Geometry check sheet. Reference: the model listing, model coordinates, mm. Face numbers are marked on the shaded views. Give positions to 0.01 mm unless a question says otherwise; leave off trailing zeros. Order: outer loops, then holes, each group sorted by start corner. A loop starts at its lowest first (then second) coordinate and runs counter-clockwise, first axis right, second up. Notation, with made-up numbers: M -24.75,24 L 23.25,24 A22 ccw 23.25,55 Z; hole C 11.25,59 d9. An arc over 180 degrees is marked long. Answer as CSV lines item,"result". Start each with the question number.
Q1. Section check A-A, the plane y = 2.7. Record the boundary of the cut face in (x, z).
Q2. Mould release check, pull along X, two halves, no side actions. Record for the marked faces 1, 2, 3 and 4: +X half, -X half, draft (parallel to the pull), parting line (faces both ways), or undercut.
Q3. Thickness scan on line 1 (X direction, y = 2.4, z = 0); line 2 (X direction, y = 2.3, z = 0); line 3 (Y direction, x = -30, z = -1.25). Record the ranges inside material, lowest first.
Q4. Section check C-C, the plane z = 0. Record the boundary of the cut face in (x, y), then the cut area to 3 significant figures.
Q5. Section check B-B, the plane x = 0. Record the boundary of the cut face in (y, z), then the cut area to 3 significant figures.
Q6. Section check D-D, the plane x = 11.5. Record the boundary of the cut face in (y, z), then the cut area to 3 significant figures.
Q7. Go/stop test with flat-tipped pins: pin 1 (1 mm diameter, centred on x = 23.5, y = 1.5, fed in from -Z); pin 2 (5 mm diameter, centred on x = 28, z = 0, fed in from -Y); pin 3 (16 mm diameter, centred on x = 0, z = 0, fed in from -Y). Record where each tip stops, or that it passes through.
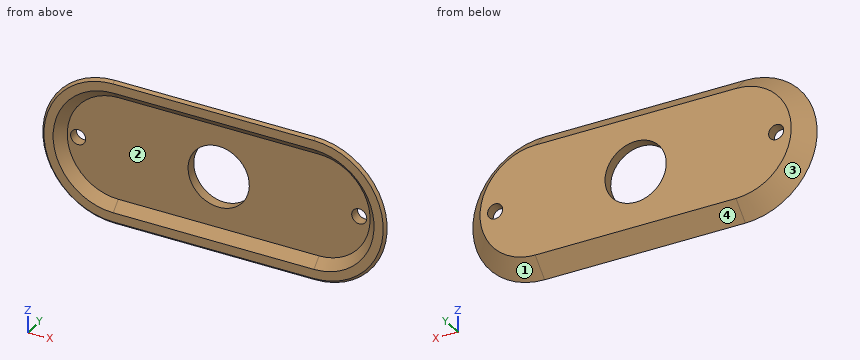
```python
from build123d import *
from OCP.BRepFilletAPI import BRepFilletAPI_MakeChamfer

# Parameters (mm, degrees)
BOSS_EXTRU_1_DEPTH      = 3.8
BOSS_EXTRU_1_TAPER      = 45
COQUE2_DEPTH            = 1.8
COQUE2_DRAFT            = 45
CHANFREIN1_SIZE         = 1
CHANFREIN1_SIZE2        = 0.707106781
ENL_V_MAT_EXTRU_1_REACH = 39.355
ESQUISSE2_R             = 1.5
ENL_V_MAT_EXTRU_2_REACH = 39.215
ESQUISSE3_R             = 6.1


# Read off the part's stored shape, not the designer's step: Coque2
with BuildPart() as part:
    # Esquisse1 → Boss.-Extru.1 (new body)
    with BuildSketch(Plane(origin=(0, 0, 0), x_dir=(1, 0, 0), z_dir=(0, 1, 0))):
        with BuildLine():
            ThreePointArc((-20, 14.8), (-34.8, 0), (-20, -14.8))
            Line((-20, -14.8), (20, -14.8))
            ThreePointArc((20, -14.8), (34.8, 0), (20, 14.8))
            Line((20, 14.8), (-20, 14.8))
        make_face()
    extrude(amount=BOSS_EXTRU_1_DEPTH, taper=BOSS_EXTRU_1_TAPER)


with BuildPart() as coque2_tool:
    # Coque2 outline → Coque2 (with draft: the straight prism first)
    with BuildSketch(Plane(origin=(0, 1.8, 0), x_dir=(1, 0, 0), z_dir=(0, 1, 0))):
        with BuildLine():
            Line((-20, -10.171572875), (20, -10.171572875))
            ThreePointArc((20, -10.171572875), (30.171572875, 0), (20, 10.171572875))
            Line((20, 10.171572875), (-20, 10.171572875))
            ThreePointArc((-20, 10.171572875), (-30.171572875, 0), (-20, -10.171572875))
        make_face()
    extrude(amount=-COQUE2_DEPTH)
    # Coque2: the draft: its side faces are tilted about the plane it starts from
    coque2_sides = [coque2_tool.faces().sort_by_distance(p)[0] for p in [
        (0, 0.9, 10.171572875),
        (30.171572875, 0.9, 0),
        (0, 0.9, -10.171572875),
        (-30.171572875, 0.9, 0),
    ]]
    draft(coque2_sides, Plane(origin=(0, 1.8, 0), x_dir=(1, 0, 0), z_dir=(0, 1, 0)), COQUE2_DRAFT)


with BuildPart() as part_1:
    add(part.part)

    # Coque2: cut by coque2_tool
    add(coque2_tool.part, mode=Mode.SUBTRACT)

    # Chanfrein1: one chamfer whose edges measure the first distance from different faces: ONE call of the kernel's chamfer builder (chamfer() names one face for all edges)
    chanfrein1_edges_1 = [part_1.edges().sort_by_distance(p)[0] for p in [
        (0, 0, -14.8),
        (0, 0, 14.8),
        (-34.8, 0, 0),
    ]]
    chanfrein1_side_1 = [part_1.faces().sort_by_distance(p)[0] for p in [
        (0, 0, -14.043672029),
    ]]
    chanfrein1_edges_2 = [part_1.edges().sort_by_distance(p)[0] for p in [
        (34.8, 0, 0),
    ]]
    chanfrein1_side_2 = [part_1.faces().sort_by_distance(p)[0] for p in [
        (32.9, 1.9, 0),
    ]]
    chanfrein1 = BRepFilletAPI_MakeChamfer(part_1.part.solid().wrapped)
    for e in chanfrein1_edges_1:
        chanfrein1.Add(CHANFREIN1_SIZE, CHANFREIN1_SIZE2, e.wrapped, chanfrein1_side_1[0].wrapped)  # the first distance lies on this face
    for e in chanfrein1_edges_2:
        chanfrein1.Add(CHANFREIN1_SIZE, CHANFREIN1_SIZE2, e.wrapped, chanfrein1_side_2[0].wrapped)  # the first distance lies on this face
    add(Compound.cast(chanfrein1.Shape()), mode=Mode.REPLACE)

    # Esquisse2 → Enlèv. mat.-Extru.1 (cut, up to next)
    with BuildSketch(Plane(origin=(0, 3.8, 0), x_dir=(1, 0, 0), z_dir=(0, 1, 0)), mode=Mode.PRIVATE) as enl_v_mat_extru_1_sk1:
        with Locations(Location((-28, 0, 0), (0, 0, 270))):
            Circle(ESQUISSE2_R)
    enl_v_mat_extru_1_tool1 = extrude(enl_v_mat_extru_1_sk1.sketch, amount=-ENL_V_MAT_EXTRU_1_REACH, mode=Mode.PRIVATE) & part_1.part
    # Esquisse2 → Enlèv. mat.-Extru.1 (cut, up to next)
    with BuildSketch(Plane(origin=(0, 3.8, 0), x_dir=(1, 0, 0), z_dir=(0, 1, 0)), mode=Mode.PRIVATE) as enl_v_mat_extru_1_sk2:
        with Locations(Location((28, 0, 0), (0, 0, 270))):
            Circle(ESQUISSE2_R)
    enl_v_mat_extru_1_tool2 = extrude(enl_v_mat_extru_1_sk2.sketch, amount=-ENL_V_MAT_EXTRU_1_REACH, mode=Mode.PRIVATE) & part_1.part
    add(enl_v_mat_extru_1_tool1.solids().sort_by_distance((-28, 3.8, 0))[0], mode=Mode.SUBTRACT)
    add(enl_v_mat_extru_1_tool2.solids().sort_by_distance((28, 3.8, 0))[0], mode=Mode.SUBTRACT)

    # Esquisse3 → Enlèv. mat.-Extru.2 (cut, up to next)
    with BuildSketch(Plane.XZ.offset(-1.8), mode=Mode.PRIVATE) as enl_v_mat_extru_2_sk1:
        with Locations(Location((0, 0, 0), (0, 0, 270))):
            Circle(ESQUISSE3_R)
    enl_v_mat_extru_2_tool1 = extrude(enl_v_mat_extru_2_sk1.sketch, amount=-ENL_V_MAT_EXTRU_2_REACH, mode=Mode.PRIVATE) & part_1.part
    add(enl_v_mat_extru_2_tool1.solids().sort_by_distance((0, 1.8, 0))[0], mode=Mode.SUBTRACT)


solid = part_1.part
```
Answer block:
1,outline,"M -20,-12.1 L 20,-12.1 A12.1 ccw 20,12.1 L -20,12.1 A12.1 ccw Z; hole C -28,0 d3; hole C 0,0 d12.2; hole C 28,0 d3"
2,face 1,"+X half"
2,face 2,"undercut"
2,face 3,"-X half"
2,face 4,"draft"
3,line 1,"x = -32.4 to -29.5, -26.5 to -6.1, 6.1 to 26.5, 29.5 to 32.4"
3,line 2,"x = -32.5 to -29.5, -26.5 to -6.1, 6.1 to 26.5, 29.5 to 32.5"
3,line 3,"y = 1.8 to 3.8"
4,outline,"M -34.3,0.5 L -33.8,0 L -31.97,0 L -30.17,1.8 L -29.5,1.8 L -29.5,3.8 L -31,3.8 Z; M -26.5,1.8 L -6.1,1.8 L -6.1,3.8 L -26.5,3.8 Z; M 6.1,1.8 L 26.5,1.8 L 26.5,3.8 L 6.1,3.8 Z; M 29.5,1.8 L 30.17,1.8 L 31.97,0 L 33.8,0 L 34.3,0.5 L 31,3.8 L 29.5,3.8 Z"
4,area,"101 mm2"
5,outline,"M 0,-13.8 L 0.5,-14.3 L 3.8,-11 L 3.8,-6.1 L 1.8,-6.1 L 1.8,-10.17 L 0,-11.97 Z; M 0,11.97 L 1.8,10.17 L 1.8,6.1 L 3.8,6.1 L 3.8,11 L 0.5,14.3 L 0,13.8 Z"
5,area,"33.3 mm2"
6,outline,"M 0,-13.8 L 0.5,-14.3 L 3.8,-11 L 3.8,11 L 0.5,14.3 L 0,13.8 L 0,11.97 L 1.8,10.17 L 1.8,-10.17 L 0,-11.97 Z"
6,area,"57.7 mm2"
7,pin 1,"stops at z = -13.36"
7,pin 2,"stops at y = 1.47"
7,pin 3,"stops at y = 1.8"
